```python
from build123d import *

# Parameters (mm, degrees)
SKETCH1_W           = 125
SKETCH1_H           = 50
BOSS_EXTRUDE1_DEPTH = 4
SKETCH2_W           = 14
SKETCH2_H           = 50
BOSS_EXTRUDE2_DEPTH = 28
SKETCH3_R           = 2.5
CUT_EXTRUDE1_DEPTH  = 4.78
SKETCH4_R           = 1.65
SKETCH4_R_2         = 3.5
CUT_EXTRUDE2_DEPTH  = 33
FILLET1_R           = 2


with BuildPart() as part:
    # Sketch1 → Boss-Extrude1 (new body)
    with BuildSketch(Plane(origin=(0, 0, 0), x_dir=(1, 0, 0), z_dir=(0, 1, 0))):
        with Locations((62.5, 25)):
            Rectangle(SKETCH1_W, SKETCH1_H)
    extrude(amount=BOSS_EXTRUDE1_DEPTH)

    # Sketch2 → Boss-Extrude2 (add)
    with BuildSketch(Plane(origin=(0, 4, 0), x_dir=(1, 0, 0), z_dir=(0, 1, 0))):
        with Locations((7, 25)):
            Rectangle(SKETCH2_W, SKETCH2_H)
        with Locations((118, 25)):
            Rectangle(SKETCH2_W, SKETCH2_H)
    extrude(amount=BOSS_EXTRUDE2_DEPTH)

    # Sketch3 → Cut-Extrude1 (cut)
    with BuildSketch(Plane.XY):
        with Locations((7, 24.5)):
            Circle(SKETCH3_R)
        with Locations((7, 10.5)):
            Circle(SKETCH3_R)
        with Locations((118, 10.5)):
            Circle(SKETCH3_R)
        with Locations((118, 24.5)):
            Circle(SKETCH3_R)
    cut_extrude1 = extrude(amount=-CUT_EXTRUDE1_DEPTH, mode=Mode.SUBTRACT)

    # Mirror1: Cut-Extrude1 across plane
    add(cut_extrude1.mirror(Plane.XY.offset(-25)), mode=Mode.SUBTRACT)

    # Sketch4 → Cut-Extrude2 (cut, through all)
    with BuildSketch(Plane.XZ):
        with Locations((82.5, -15)):
            Circle(SKETCH4_R)
        with Locations((42.5, -15)):
            Circle(SKETCH4_R)
        with Locations((82.5, -35)):
            Circle(SKETCH4_R)
        with Locations((42.5, -35)):
            Circle(SKETCH4_R)
        with Locations((37.5, -25)):
            Circle(SKETCH4_R_2)
        with Locations((87.5, -25)):
            Circle(SKETCH4_R_2)
    extrude(amount=-CUT_EXTRUDE2_DEPTH, mode=Mode.SUBTRACT)

    # Fillet1
    fillet1_edges = [part.edges().sort_by_distance(p)[0] for p in [
        (125, 0, -25),
        (0, 0, -25),
    ]]
    fillet(fillet1_edges, radius=FILLET1_R)


solid = part.part
```
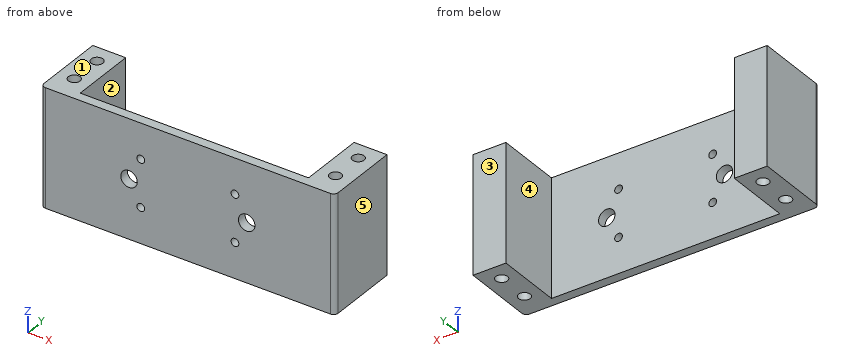
Can you work these out from the model? Positions are in its coordinate system, mm. Face numbers are marked on the shaded views. A direction names the side the tool comes from. Give positions to 0.01 mm unless a question says otherwise; leave off trailing zeros. Write each loop counter-clockwise with the first axis right and the second up, starting at its lowest first coordinate (ties: lowest second). Pieces come first, ordered by that corner, then holes. Notation, with made-up numbers: (35.25, 52.25) -> (42.25, 52.25) arc R13 ccw to (42.25, 57.25) -> close; hole circle Ø2 at (87, 69.25). An arc over 180 degrees is marked (long way). Write item = value, one per line.
(1) I need wall thicknesses on probe 1 along Y at (x, z) = (118, -3.4); probe 2 along Z at (x, y) = (42.5, 1.4); probe 3 along X at (y, z) = (11, -24). Which ranges of each line are inside material? Lowest first, please. Write a range as from..to.
Worked out:
probe_1 = 0..8, 13..22, 27..32
probe_2 = -50..-36.65, -33.35..-16.65, -13.35..0
probe_3 = 0..14, 111..125
(2) Suppose I cut it at C-C on y = 10.5. Write out the boundary of the cut face in (x, z), then the cut area to 3 significant figures.
Worked out:
outline = (0, -50) -> (4.5, -50) -> (4.5, -45.22) -> (9.5, -45.22) -> (9.5, -50) -> (14, -50) -> (14, 0) -> (9.5, 0) -> (9.5, -4.78) -> (4.5, -4.78) -> (4.5, 0) -> (0, 0) -> close; (111, -50) -> (115.5, -50) -> (115.5, -45.22) -> (120.5, -45.22) -> (120.5, -50) -> (125, -50) -> (125, 0) -> (120.5, 0) -> (120.5, -4.78) -> (115.5, -4.78) -> (115.5, 0) -> (111, 0) -> close
area = 1,300 mm^2
(3) Suppose I cut it at B-B on z = -25. Write out the boundary of the cut face in (x, y), then the cut area to 3 significant figures.
Worked out:
outline = (0, 2) arc R2 ccw to (2, 0) -> (34, 0) -> (34, 4) -> (14, 4) -> (14, 32) -> (0, 32) -> close; (41, 0) -> (84, 0) -> (84, 4) -> (41, 4) -> close; (91, 0) -> (123, 0) arc R2 ccw to (125, 2) -> (125, 32) -> (111, 32) -> (111, 4) -> (91, 4) -> close
area = 1,230 mm^2
(4) Suppose I cut it at D-D on z = -3.5. Write out the boundary of the cut face in (x, y), then the cut area to 3 significant figures.
Worked out:
outline = (0, 2) arc R2 ccw to (2, 0) -> (123, 0) arc R2 ccw to (125, 2) -> (125, 32) -> (111, 32) -> (111, 4) -> (14, 4) -> (14, 32) -> (0, 32) -> close; hole circle Ø5 at (7, 10.5); hole circle Ø5 at (7, 24.5); hole circle Ø5 at (118, 10.5); hole circle Ø5 at (118, 24.5)
area = 1,200 mm^2
(5) Thinking about a two-plate mould opening in X: for the marked faces 3, 4 and 5, which applies, released by +X, released by -X, zero draft, split by the parting line, or undercut?
Worked out:
face_3 = zero draft
face_4 = undercut
face_5 = released by +X
(6) For the marked faces 1 and 2, which set-ups out of +Z, -Z, +X, -X, +Y, -Y let a thin tool reach every point of the face, with its end or its side?
Worked out:
face_1 = +Z, +X, -X, +Y, -Y
face_2 = +Z, -Z, +Y
(7) I'm going to push flat-ended pins straight in: P1, Ø2.5, axis at x = 118.5, y = 11.5, coming from the -Z side; P2, Ø8, axis at x = 37.5, z = -25, coming from the +Y side. Where does each tip first touch, or does it pass through?
Worked out:
P1 = -45.22
P2 = 4
(8) Suppose I cut it at A-A on x = 82.5. Write out the boundary of the cut face in (y, z).
Worked out:
outline = (0, -50) -> (4, -50) -> (4, -36.65) -> (0, -36.65) -> close; (0, -33.35) -> (4, -33.35) -> (4, -16.65) -> (0, -16.65) -> close; (0, -13.35) -> (4, -13.35) -> (4, 0) -> (0, 0) -> close
